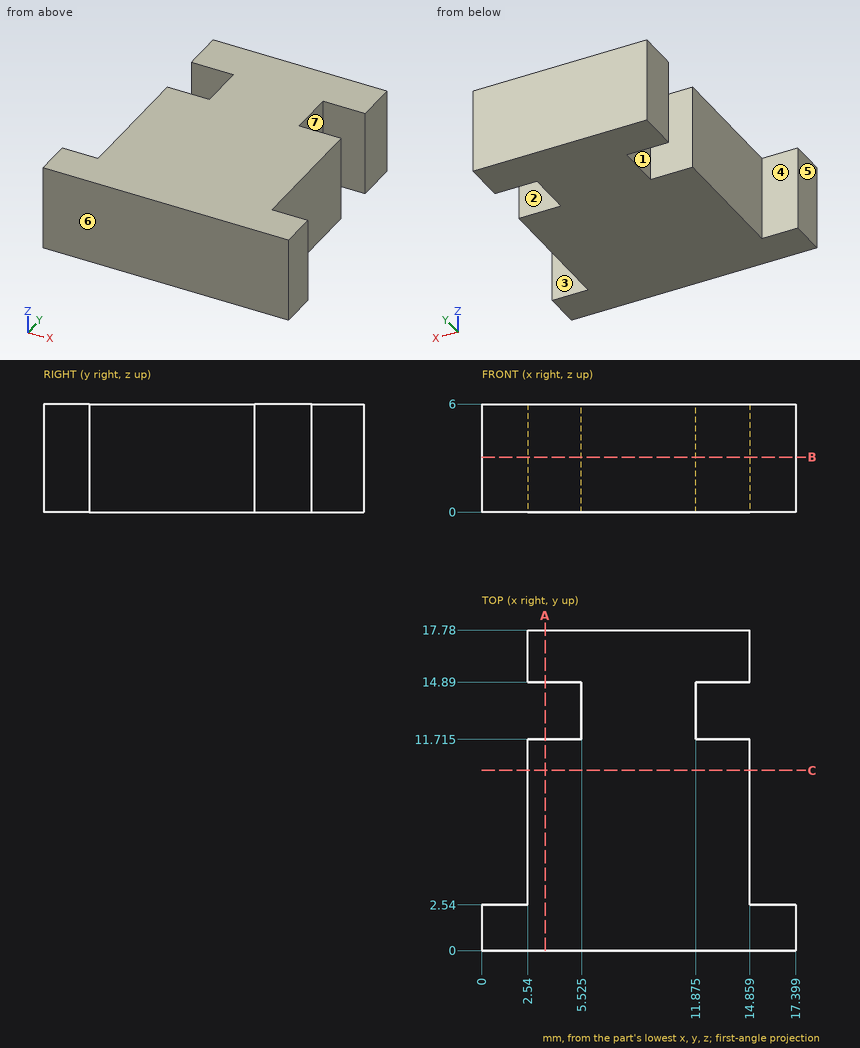
Verification items for this drawing (mm, ordinates from the low corner). A direction names the side the tool comes from. Coordinates: 2 decimals unless noted, no trailing zeros. Write each loop counter-clockwise with the first axis right and the second up, starting at its lowest first coordinate (ties: lowest second). Pieces come first, ordered by that corner, then holes. Notation, with made-up numbers: M 72,13.25 L 97,13.25 A24 cw 97,27.25 Z; hole C 70,65.25 d1. An arc over 180 degrees is marked long. Use one line per item in the form item = value. Start each with the question number.
1) Release check for a two-part mould opening along Y. For the marked faces 5, 6 and 7 record: pulls with the +Y half, pulls with the -Y half, needs draft (parallel to the pull), parting line crosses it, or undercut.
2) Section check C-C on y = 10. Enter the section's corners in (x, z).
3) Thickness scan on probe 1 along Y at (x, z) = (12.5, 1) (1 decimal); probe 2 along X at (y, z) = (5.25, 0.5); probe 3 along Y at (x, z) = (16.75, 5.45). Record the ranges inside material, lowest first. Write a range as from..to.
4) Section check A-A on x = 3.5. Enter the section's corners in (y, z) (1 decimal).
5) Go/stop test with flat-tipped pins: pin 1 Ø0.8 at (x, z) = (1, 2) entering from +Y; pin 2 Ø3 at (y, z) = (16, 3) entering from +X; pin 3 Ø2.5 at (y, z) = (16, 2.5) entering from -X. Record where each tip stops, or that it passes through.
6) Set-up check for the marked faces 1, 2, 3 and 4: record each of +Z, -Z, +X, -X, +Y, -Y from which the full face is reachable in a straight line by a thin tool's end or side.
7) Section check B-B on z = 3.05. Enter the section's corners in (x, y) (1 decimal).
Responses:
q1.face_5 = needs draft
q1.face_6 = pulls with the -Y half
q1.face_7 = undercut
q2.outline = M 2.54,0 L 14.86,0 L 14.86,6 L 2.54,6 Z
q3.probe_1 = 0..11.7, 14.9..17.8
q3.probe_2 = 2.54..14.86
q3.probe_3 = 0..2.54
q4.outline = M 0,0 L 11.7,0 L 11.7,6 L 0,6 Z; M 14.9,0 L 17.8,0 L 17.8,6 L 14.9,6 Z
q5.pin_1 = 2.54
q5.pin_2 = 14.86
q5.pin_3 = 2.54
q6.face_1 = +Z, -Z, -X
q6.face_2 = +Z, -Z, +X
q6.face_3 = +Z, -Z, +X, +Y
q6.face_4 = +Z, -Z, -X, +Y
q7.outline = M 0,0 L 17.4,0 L 17.4,2.5 L 14.9,2.5 L 14.9,11.7 L 11.9,11.7 L 11.9,14.9 L 14.9,14.9 L 14.9,17.8 L 2.5,17.8 L 2.5,14.9 L 5.5,14.9 L 5.5,11.7 L 2.5,11.7 L 2.5,2.5 L 0,2.5 Z
